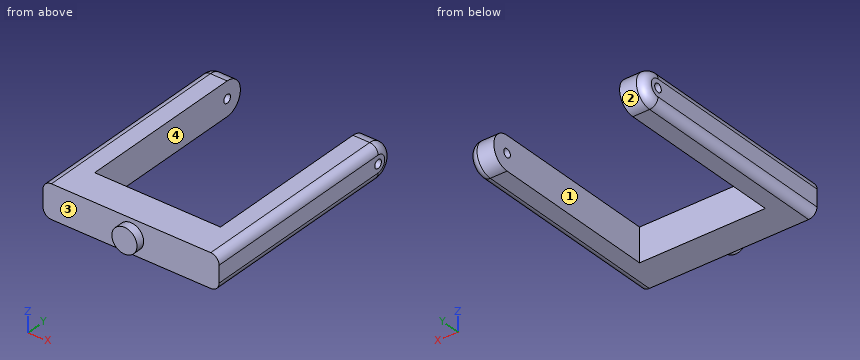
Autodesk Inventor part; units mm, degrees
ref_plane "YZ Plane" through (0, 0, 0) normal (1, 0, 0) x (0, 1, 0)
ref_plane "XZ Plane" through (0, 0, 0) normal (0, 1, 0) x (-1, 0, 0)
ref_plane "XY Plane" through (0, 0, 0) normal (0, 0, 1) x (1, 0, 0)
sketch "Sketch1" plane through (0, 0, 0) normal (1, 0, 0) x (0, 1, 0)
  line L0 (0, 20) -> (40, 20)
  line L1 (40, 20) -> (40, -20)
  line L2 (40, -20) -> (0, -20)
  line L3 (0, -20) -> (0, 20)
  point P0 (0, 0)
  dimension "d0" = 20
  dimension "d1" = 40
  dimension "d2" = 40
  dimension "d3" = 40
extrude "Extrusion1" add sketch "Sketch1" along normal mid plane 210
sketch "Sketch2" plane through (-105, 40, 20) normal (0, 1, 0) x (1, 0, 0)
  line L0 (210, 40) -> (210, 0)
  line L1 (0, 40) -> (210, 40)
  line L2 (210, 0) -> (180, 0)
  line L3 (180, 0) -> (180, 40)
  line L4 (180, 40) -> (210, 40)
  line L5 (210, 40) -> (210, 0)
  line L6 (0, 0) -> (210, 0)
  line L7 (0, 0) -> (30, 0)
  line L8 (30, 0) -> (30, 40)
  line L9 (30, 40) -> (0, 40)
  line L10 (0, 40) -> (0, 0)
  point P0 (105, 20)
  point P1 (0, 40)
  point P2 (30, 0)
  point P3 (30, 40)
  dimension "d6" = 30
  dimension "d7" = 30
extrude "Extrusion2" add sketch "Sketch2" along normal blind 200 contours L0 L2 L3 L1 | L8 L6 L10 L1
sketch "Sketch3" plane through (-75, 40, 20) normal (1, 0, 0) x (0, 0, -1)
  line L0 (40, 200) -> (0, 200)
  circle A0 centre (20, 200) radius 20
  circle A1 centre (20, 200) radius 5
  point P0 (20, -40)
  dimension "d14" = 10
extrude "Extrusion3" add sketch "Sketch3" against normal up to surface (30 mm away)
sketch "Sketch4" plane through (105, 0, 0) normal (1, 0, 0) x (0, 0, -1)
  arc A0 (20, 240) -> (-20, 240) centre (0, 240) ccw
  line L0 (-20, 240) -> (20, 240)
  circle A1 centre (0, 240) radius 20
  point P0 (0, 0)
  point P1 (-20, 240)
extrude "Extrusion4" add sketch "Sketch4" against normal up to surface (30 mm away)
sketch "Sketch5" plane through (105, 0, 0) normal (1, 0, 0) x (0, 0, -1)
  arc A0 (20, 240) -> (-20, 240) centre (0, 240) ccw
  circle A1 centre (0, 240) radius 5
  point P0 (0, 0)
  dimension "d15" = 10
extrude "Extrusion5" cut sketch "Sketch5" against normal through all
fillet "Fillet1" radius 10 6 edges at (105, 120, 20) (105, 120, -20) (105, 260, 0) (-105, 120, -20) (-105, 120, 20) (-105, 260, 0)
sketch "Sketch6" plane through (-95, 0, -20) normal (0, -1, 0) x (1, 0, 0)
  circle A0 centre (95, 20) radius 15
  dimension "d21" = 30
extrude "Extrusion6" add sketch "Sketch6" along normal blind 10
properties part number "AERO - Fork"
Geometry check sheet. Reference: the model listing, model coordinates, mm. Face numbers are marked on the shaded views. A direction names the side the tool comes from. Coordinates: 2 decimals unless noted, no trailing zeros. Order: outer loops, then holes, each group sorted by start corner. A loop starts at its lowest first (then second) coordinate and runs counter-clockwise, first axis right, second up.
Q1. Sectioned sample at C-C on x = 0. Record the cut outline in (y, z), and give its area (3 significant figures).
Reply:
outline: (-10, -15) - (0, -15) - (0, -20) - (40, -20) - (40, 20) - (0, 20) - (0, 15) - (-10, 15) - close
area: 1,900 mm2
Q2. Depth check by flat-ended pin: pin 1 Ø5 at (x, z) = (-62.5, -15.5) entering from +Y; pin 2 Ø5 at (x, z) = (-79.5, 8.5) entering from -Y; pin 3 Ø6 at (y, z) = (240, 0) entering from +X. Enter the tip coordinate at first touch or a pass-through.
Reply:
pin 1: stops at y = 40
pin 2: stops at y = 0
pin 3: passes through
Q3. Thickness scan on probe 1 along X at (y, z) = (117.5, 8.5); probe 2 along Y at (x, z) = (-83, 0); probe 3 along X at (y, z) = (156.5, -17). Record the ranges inside material, lowest first.
Reply:
probe 1: x = -105 to -75, 75 to 105
probe 2: y = 0 to 235, 245 to 260
probe 3: x = -102.14 to -75, 75 to 102.14
Q4. Tool access check on the marked faces 1 and 2. Record the directions out of +Z, -Z, +X, -X, +Y, -Y that give a thin tool (end or side, any length) a straight path to the whole face; none if there is none.
Reply:
face 1: +Z, -Z, +Y
face 2: +X, -X, +Y
Q5. Sectioned sample at A-A on y = 104. Record the cut outline in (x, z).
Reply:
outline: (-105, -10) arc R10 ccw to (-95, -20) - (-75, -20) - (-75, 20) - (-95, 20) arc R10 ccw to (-105, 10) - close; (75, -20) - (95, -20) arc R10 ccw to (105, -10) - (105, 10) arc R10 ccw to (95, 20) - (75, 20) - close
Q6. Sectioned sample at B-B on z = 0. Give the number of separate pieces and of enclosed holes in the cut face, and give its area (3 significant figures).
Reply:
separate pieces: 3
enclosed holes: 0
area: 21,300 mm2
Q7. Draft check along X on the marked faces 3 and 4. Enter one of: released by +X, released by -X, zero draft, split by the parting line, or undercut.
Reply:
face 3: zero draft
face 4: undercut
